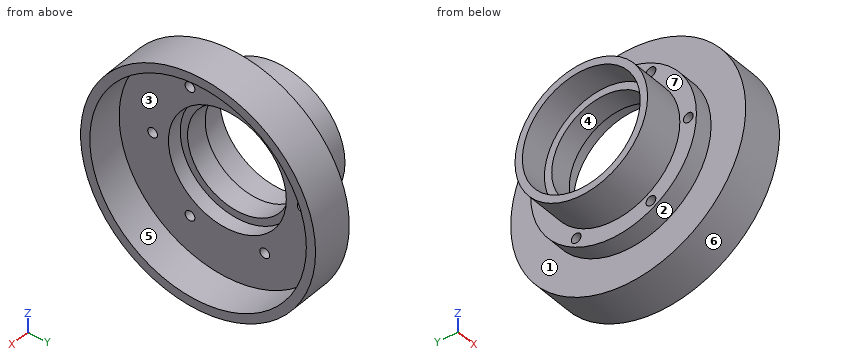
Solid Edge part; units mm, degrees
sketch "Sketch1" plane through (0, 0, 0) normal (0, 0, 1) x (1, 0, 0)
  line L0 (20, 58.79) -> (0, 58.79)
  line L1 (0, 58.79) -> (0, 32)
  line L2 (0, 32) -> (-8, 32)
  line L3 (-8, 32) -> (-8, 28)
  line L4 (-8, 28) -> (-20, 28)
  line L5 (-20, 28) -> (-20, 32)
  line L6 (-20, 32) -> (-35, 32)
  line L7 (-35, 32) -> (-35, 36)
  line L8 (-35, 36) -> (-3, 36)
  line L9 (-3, 36) -> (-3, 63.79)
  line L10 (-3, 63.79) -> (20, 63.79)
  line L11 (20, 63.79) -> (20, 58.79)
  dimension "D1" = 3
  dimension "D2" = 20
  dimension "D3" = 8
  dimension "D4" = 20
  dimension "D5" = 35
  dimension "D6" = 35
  dimension "D7" = 3
  dimension "D8" = 20
  dimension "D9" = 20
revolve "RevolvedProtrusion1" add sketch "Sketch1" angle 360 about axis through (0, 0, 0) along (1, 0, 0)
sketch "Sketch2" plane through (-3, 0, 0) normal (-1, 0, 0) x (0, -1, 0)
  circle A0 centre (0, 0) radius 45
  circle A1 centre (0, 0) radius 36
extrude "ExtrudedProtrusion_1" add sketch "Sketch2" along normal blind 10
hole "Hole_2" at (-13, 40.6134, 0) direction (1, 0, 0) diameter 5.3 end up to next
hole "Hole1" at (-13, 20.3067, 35.1723) direction (1, 0, 0) diameter 5.3 end up to next
hole "Hole2" at (-13, -20.3067, 35.1723) direction (1, 0, 0) diameter 5.3 end up to next
hole "Hole3" at (-13, -40.6134, 0) direction (1, 0, 0) diameter 5.3 end up to next
hole "Hole4" at (-13, -20.3067, -35.1723) direction (1, 0, 0) diameter 5.3 end up to next
hole "Hole5" at (-13, 20.3067, -35.1723) direction (1, 0, 0) diameter 5.3 end up to next
properties material "Aluminum, 6061-T6"
Verification items for the finished model (mm, model axes). Face numbers are marked on the shaded views. A direction names the side the tool comes from. Coordinates: 2 decimals unless noted, no trailing zeros. Write each loop counter-clockwise with the first axis right and the second up, starting at its lowest first coordinate (ties: lowest second). Pieces come first, ordered by that corner, then holes. Notation, with made-up numbers: (85.5, 77.5) -> (98.5, 77.5) arc R18 ccw to (98.5, 111.5) -> close; hole circle Ø10 at (44, 61). An arc over 180 degrees is marked (long way). One line per item, written item: value. Start each with the question number.
Q1. Cross-section at A-A on y = 5. Enter the section's corners in (x, z), and give its area (3 significant figures).
Q2. Cross-section at C-C on z = 0. State how many separate pieces and enclosed holes the cut face has, and give its area (3 significant figures).
Q3. Cross-section at B-B on z = 26. Enter the section's corners in (x, y).
Q4. Cross-section at D-D on x = 2. Enter the section's corners in (y, z), and give its area (3 significant figures).
Q5. Access from +Z, -Z, +X, -X, +Y, -Y to the whole of each face (thin tool, end or side, straight path). Record for the marked faces 5, 6 and 7.
Q6. Thickness scan on L1, parallel to Z at x = -7.5, y = -18; L2, parallel to Y at x = 9, z = -0.5; L3, parallel to X at y = -20, z = -52. Record the ranges inside material, lowest first. Write a range as from..to.
Q7. Go/stop test with flat-tipped pins: P1, Ø4, axis at y = 40.61, z = 0, coming from the -X side (3 decimals); P2, Ø12, axis at x = -29.5, y = 14.5, coming from the -Z side; P3, Ø8.5, axis at y = 20.31, z = 35.17, coming from the -X side; P4, Ø1.5, axis at x = 4, y = -49.5, coming from the -Z side. Record where each tip stops, or that it passes through.
Q8. Mould release check, pull along Z, two halves, no side actions. Record for the marked faces 1, 2, 3 and 4: pulls with the +Z half, pulls with the -Z half, needs draft (parallel to the pull), parting line crosses it, or undercut.
Checked values:
1. outline: (-35, -35.65) -> (-13, -35.65) -> (-13, -44.72) -> (-3, -44.72) -> (-3, -63.59) -> (20, -63.59) -> (20, -58.58) -> (0, -58.58) -> (0, -31.61) -> (-8, -31.61) -> (-8, -27.55) -> (-20, -27.55) -> (-20, -31.61) -> (-35, -31.61) -> close; (-35, 31.61) -> (-20, 31.61) -> (-20, 27.55) -> (-8, 27.55) -> (-8, 31.61) -> (0, 31.61) -> (0, 58.58) -> (20, 58.58) -> (20, 63.59) -> (-3, 63.59) -> (-3, 44.72) -> (-13, 44.72) -> (-13, 35.65) -> (-35, 35.65) -> close
1. area: 930 mm²
2. separate pieces: 4
2. enclosed holes: 0
2. area: 785 mm²
3. outline: (-35, -24.9) -> (-13, -24.9) -> (-13, -36.73) -> (-3, -36.73) -> (-3, -58.25) -> (20, -58.25) -> (20, -52.73) -> (0, -52.73) -> (0, -18.65) -> (-8, -18.65) -> (-8, -10.39) -> (-20, -10.39) -> (-20, -18.65) -> (-35, -18.65) -> close; (-35, 18.65) -> (-20, 18.65) -> (-20, 10.39) -> (-8, 10.39) -> (-8, 18.65) -> (0, 18.65) -> (0, 52.73) -> (20, 52.73) -> (20, 58.25) -> (-3, 58.25) -> (-3, 36.73) -> (-13, 36.73) -> (-13, 24.9) -> (-35, 24.9) -> close
4. outline: circle Ø127.58 at (0, 0); hole circle Ø117.58 at (0, 0)
4. area: 1,930 mm²
5. face 5: +X
5. face 6: +X, -X
5. face 7: -X
6. L1: z = -41.24..-36.48, -33.87..-26.46, 26.46..33.87, 36.48..41.24
6. L2: y = -63.79..-58.79, 58.79..63.79
6. L3: x = -3..0
7. P1: passes through
7. P2: stops at z = -34.98
7. P3: stops at x = -13
7. P4: stops at z = -41.14
8. face 1: needs draft
8. face 2: parting line crosses it
8. face 3: undercut
8. face 4: undercut
